Could you check a few things on this model? Use its own coordinates, in mm. A direction names the side the tool comes from. Give positions to 0.01 mm unless a question says otherwise; leave off trailing zeros. Order: outer loops, then holes, each group sorted by start corner. A loop starts at its lowest first (then second) coordinate and runs counter-clockwise, first axis right, second up.
(1) Will these pins go through, and if not, where does the flat tip stop? pin 1 (5 mm diameter, centred on y = 20, z = -30, fed in from +X); pin 2 (3 mm diameter, centred on x = 5, z = -5, fed in from +Y); pin 3 (2 mm diameter, centred on x = -5.5, y = 29.5, fed in from +Z).
(2) Imagine slicing it at C-C, the plane x = 22. Write out the boundary of the cut face in (y, z), then the cut area to 3 significant figures.
(3) If we mould it in two halves opening along Y, with no side actions, what happens to faces 1 (the flat face through (10, 22, -6)), 2 (the cylindrical face through (5.96, 37.69, 0.99)), 3 (the flat face through (19, 45, 1)), 4 (the cylindrical face through (29.89, 38.66, 0.99))? For each: released by +Y, released by -Y, zero draft, split by the parting line, or undercut.
(4) Imagine slicing it at A-A, the plane y = 6.5. Write out the boundary of the cut face in (x, z).
(5) Imagine slicing it at B-B, the plane x = 32. Write out the boundary of the cut face in (y, z), then the cut area to 3 significant figures.
(6) If I drill on probe 1 along Y at (x, z) = (5, 1.4); probe 2 along X at (y, z) = (40, 1.05); probe 3 along Y at (x, z) = (10, -35), over which ranges is the centre line in solid material (lowest first)?
(7) Imagine slicing it at D-D, the plane y = 27. Write out the boundary of the cut face in (x, z), then the cut area to 3 significant figures.
(8) On a 3-axis mill with a long thin cutter (end or side, diameter ignored), from which of +Z, -Z, +X, -X, +Y, -Y can I reach the whole of each face in a straight line? I mean faces 5 (the cylindrical face through (34.11, 6.34, 0.99)), 6 (the flat face through (5, 9, -30)), 7 (the flat face through (0, 22, -3)), 8 (the flat face through (5, 36, -30)). Say none if no direction works.
Autodesk Fusion 360 part; units mm, degrees
sketch "Sketch1" plane through (0, 0, 0) normal (0, 0, 1) x (1, 0, 0)
  line L0 (0, 0) -> (37, 0)
  line L1 (37, 0) -> (37, 45)
  line L2 (37, 45) -> (0, 45)
  line L3 (0, 45) -> (0, 0)
  dimension "d1" = 37
  dimension "d2" = 45
extrude "Extrude1" add sketch "Sketch1" along normal blind 2
sketch "Sketch2" plane through (0, 0, 2) normal (0, 0, 1) x (-1, 0, 0)
  line L0 (0, -45) -> (0, 0)
  line L1 (0, 0) -> (-37, 0)
  line L2 (-37, 0) -> (-37, -45)
  line L3 (-37, -45) -> (0, -45)
sketch "Sketch3" plane through (0, 0, 2) normal (0, 0, 1) x (-1, 0, 0)
sketch "Sketch4" plane through (0, 0, 2) normal (0, 0, 1) x (-1, 0, 0)
  point P0 (-5, -40)
hole "Hole1" at (5, 40, 2) direction (0, 0, -1) diameter 5 depth 15 tip angle 180
ref_plane "WorkPlane1" through (18.5, 22.5, 1) normal (1, 0, 0) x (0, 1, 0)
ref_plane "WorkPlane2" through (18.5, 22.5, 1) normal (0, -1, 0) x (1, 0, 0)
mirror "Mirror1" about plane through (18.5, 22.5, 1) normal (1, 0, 0) of "Hole1"
mirror "Mirror2" about plane through (18.5, 22.5, 1) normal (0, -1, 0) of "Hole1", "Mirror1"
sketch "Sketch5" plane through (0, 0, 0) normal (0, 0, -1) x (1, 0, 0)
  circle A0 centre (32, -5) radius 2.5
  circle A1 centre (5, -5) radius 2.5
  circle A2 centre (32, -40) radius 2.5
  circle A3 centre (5, -40) radius 2.5
  line L0 (0, 0) -> (0, -45)
  line L1 (0, -45) -> (37, -45)
  line L2 (37, -45) -> (37, 0)
  line L3 (37, 0) -> (0, 0)
  line L4 (0, -15) -> (10, -15)
  line L5 (10, -15) -> (10, -25)
  line L6 (10, -25) -> (0, -25)
  line L7 (0, -25) -> (0, -15)
extrude "Extrude2" add sketch "Sketch5" along normal blind 35 contours L0 L4 L5 L6 L7
sketch "Sketch6" plane through (0, 15, 0) normal (0, -1, 0) x (1, 0, 0)
  line L0 (10, 0) -> (0, 0)
  line L1 (0, 0) -> (0, -35)
  line L2 (0, -35) -> (10, -35)
  line L3 (10, -35) -> (10, 0)
  point P0 (0, -30)
sketch "Sketch7" plane through (0, 15, 0) normal (0, -1, 0) x (1, 0, 0)
sketch "Sketch8" plane through (0, 15, 0) normal (0, -1, 0) x (1, 0, 0)
  circle A0 centre (5, -30) radius 18.5
  dimension "d14" = 37
extrude "Extrude3" add sketch "Sketch8" against normal blind 16
extrude "Extrude4" add 1 faces at (3.6278, 31, -23.9879) along direction (0, -1, 0) blind 22
extrude "Extrude5" add 1 faces at (5, 25, -3.8333) along direction (0, 1, 0) blind 5
extrude "Extrude6" add 1 faces at (3.6278, 31, -23.9879) along direction (0, 1, 0) blind 5
Answer block:
1. pin 1: stops at x = 23.5
1. pin 2: stops at y = 30
1. pin 3: stops at z = -14.13
2. outline: (0, 0) - (45, 0) - (45, 2) - (0, 2) - close; (9, -37.3) - (36, -37.3) - (36, -22.7) - (9, -22.7) - close
2. area: 484 mm2
3. face 1: zero draft
3. face 2: undercut
3. face 3: released by +Y
3. face 4: undercut
4. outline: (0, 0) - (3, 0) - (3, 2) - (0, 2) - close; (7, 0) - (30, 0) - (30, 2) - (7, 2) - close; (34, 0) - (37, 0) - (37, 2) - (34, 2) - close
5. outline: (0, 0) - (2.5, 0) - (2.5, 2) - (0, 2) - close; (7.5, 0) - (37.5, 0) - (37.5, 2) - (7.5, 2) - close; (42.5, 0) - (45, 0) - (45, 2) - (42.5, 2) - close
5. area: 70.0 mm2
6. probe 1: y = 0 to 2.5, 7.5 to 37.5, 42.5 to 45
6. probe 2: x = 0 to 2.5, 7.5 to 29.5, 34.5 to 37
6. probe 3: y = 9 to 36
7. outline: (0, -12.19) arc R18.5 ccw (long way) to (10, -12.19) - (10, 0) - (37, 0) - (37, 2) - (0, 2) - close
7. area: 1,270 mm2
8. face 5: +Z, -Z
8. face 6: -Z, +X, -X, -Y
8. face 7: +Z, -X, +Y, -Y
8. face 8: -Z, +X, -X, +Y
